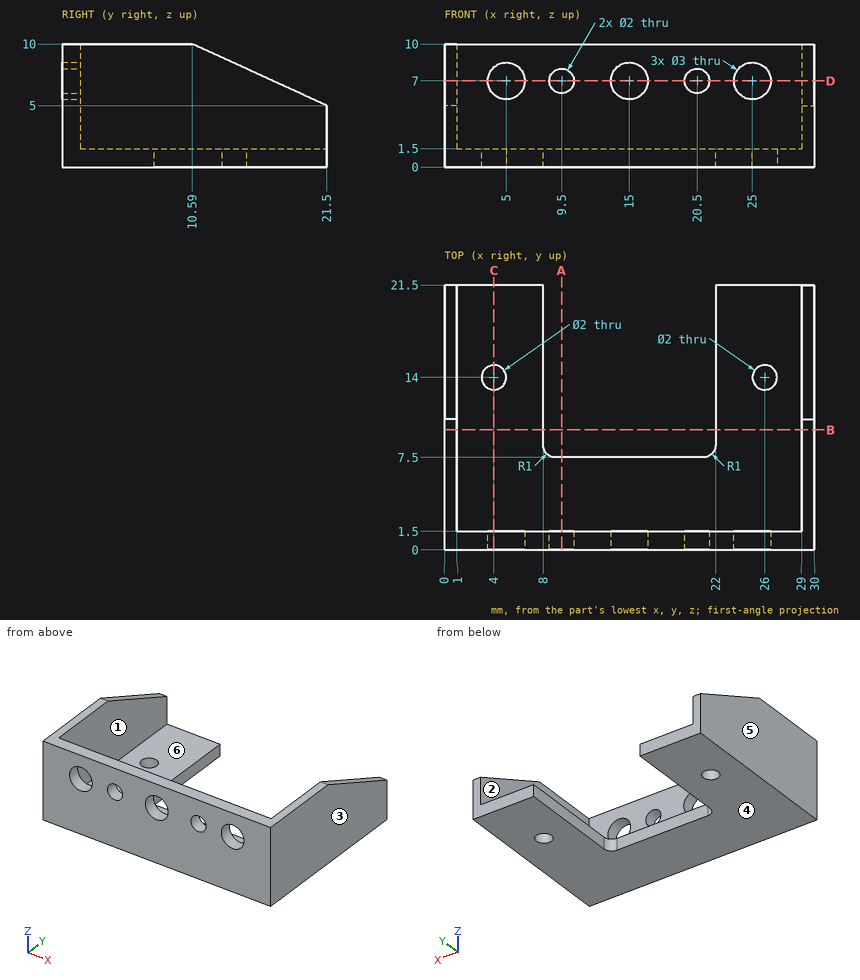
Can you work these out from the drawing? Everything is in mm from the part's minimum corner. A direction names the side the tool comes from. Coordinates: 2 decimals unless noted, no trailing zeros. Loops run counter-clockwise (first coordinate to the right, second up) from the corner with the lowest first, then second, coordinate; pieces in that order, holes last. Notation, with made-up numbers: (49.25, 26.5) -> (66.25, 26.5) arc R27 cw to (66.25, 52.5) -> close; hole circle Ø5 at (62.5, 21.25). An arc over 180 degrees is marked (long way). Return JSON: item names as keys, results as strings.
1) If we section it at A-A, the plane x = 9.5: Write out the boundary of the cut face in (y, z).
Results below:
{"outline": "(0, 0) -> (7.5, 0) -> (7.5, 1.5) -> (1.5, 1.5) -> (1.5, 6) -> (0, 6) -> close; (0, 8) -> (1.5, 8) -> (1.5, 10) -> (0, 10) -> close"}
2) Will these pins go through, and if not, where does the flat tip stop? pin 1 (10 mm diameter, centred on x = 12.5, y = 14, fed in from +Z); pin 2 (1.2 mm diameter, centred on x = 4, y = 14, fed in from -Z); pin 3 (2.5 mm diameter, centred on x = 9.5, z = 7, fed in from +Y).
Results below:
{"pin 1": "z = 1.5", "pin 2": "through", "pin 3": "y = 1.5"}
3) I need wall thicknesses on line 1 (X direction, y = 1.05, z = 7); line 2 (Z direction, x = 15, y = 0.3); line 3 (X direction, y = 14, z = 2.5). Which ranges of each line are inside material? Lowest first, please. Write a range as from..to.
Results below:
{"line 1": "0..3.5, 6.5..8.5, 10.5..13.5, 16.5..19.5, 21.5..23.5, 26.5..30", "line 2": "0..5.5, 8.5..10", "line 3": "0..1, 29..30"}
4) If we section it at C-C, the plane x = 4: Write out the boundary of the cut face in (y, z).
Results below:
{"outline": "(0, 0) -> (13, 0) -> (13, 1.5) -> (1.5, 1.5) -> (1.5, 5.88) -> (0, 5.88) -> close; (0, 8.12) -> (1.5, 8.12) -> (1.5, 10) -> (0, 10) -> close; (15, 0) -> (21.5, 0) -> (21.5, 1.5) -> (15, 1.5) -> close"}
5) If we section it at B-B, the plane y = 9.75: Write out the boundary of the cut face in (x, z), then the cut area to 3 significant figures.
Results below:
{"outline": "(0, 0) -> (8, 0) -> (8, 1.5) -> (1, 1.5) -> (1, 10) -> (0, 10) -> close; (22, 0) -> (30, 0) -> (30, 10) -> (29, 10) -> (29, 1.5) -> (22, 1.5) -> close", "area": "41.0 mm²"}
6) Thinking about a two-plate mould opening in X: for the marked faces 1, 2, 3 and 4, which applies, +X half, -X half, draft (parallel to the pull), parting line (faces both ways), or undercut?
Results below:
{"face 1": "undercut", "face 2": "undercut", "face 3": "+X half", "face 4": "draft"}
7) For the marked faces 5 and 6, which set-ups out of +Z, -Z, +X, -X, +Y, -Y let a thin tool reach every point of the face, with its end or its side?
Results below:
{"face 5": "+Z, -Z, -X, +Y, -Y", "face 6": "+Z, +Y"}
8) If we section it at D-D, the plane z = 7: Write out the boundary of the cut face in (x, y), then the cut area to 3 significant figures.
Results below:
{"outline": "(0, 0) -> (3.5, 0) -> (3.5, 1.5) -> (1, 1.5) -> (1, 17.14) -> (0, 17.14) -> close; (6.5, 0) -> (8.5, 0) -> (8.5, 1.5) -> (6.5, 1.5) -> close; (10.5, 0) -> (13.5, 0) -> (13.5, 1.5) -> (10.5, 1.5) -> close; (16.5, 0) -> (19.5, 0) -> (19.5, 1.5) -> (16.5, 1.5) -> close; (21.5, 0) -> (23.5, 0) -> (23.5, 1.5) -> (21.5, 1.5) -> close; (26.5, 0) -> (30, 0) -> (30, 17.14) -> (29, 17.14) -> (29, 1.5) -> (26.5, 1.5) -> close", "area": "56.8 mm²"}
